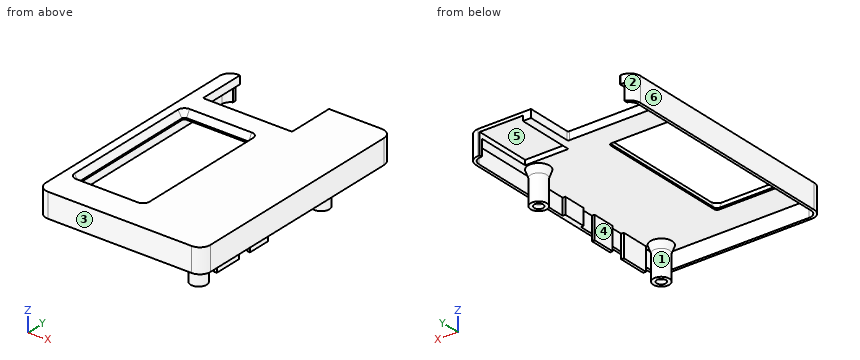
```python
from build123d import *
from OCP.BRepFilletAPI import BRepFilletAPI_MakeChamfer

# Parameters (mm, degrees)
SKETCH_1_W          = 61
SKETCH_1_H          = 90
EXTRUDE_1_DEPTH     = 3
SKETCH_3_W          = 25
SKETCH_3_H          = 51
CUT_EXTRUDE_1_DEPTH = 3
FILLET_1_R          = 1
CHAMFER_1_SIZE      = 1.4
CHAMFER_1_SIZE2     = 2.424871131
SKETCH_7_R          = 3
EXTRUDE_2_DEPTH     = 12.2
CHAMFER_2_SIZE      = 1
CHAMFER_2_SIZE2     = 2.747477419
SKETCH_8_R          = 1.3
CUT_EXTRUDE_2_DEPTH = 6
CHAMFER_3_SIZE      = 0.4
CHAMFER_3_SIZE2     = 1.098990968
SKETCH_10_W         = 1
SKETCH_10_H         = 10.4
SKETCH_10_H_2       = 8.6
EXTRUDE_3_DEPTH     = 8.5
SKETCH_11_W         = 61
SKETCH_11_H         = 90
SKETCH_11_W_2       = 59
SKETCH_11_H_2       = 88
EXTRUDE_4_DEPTH     = 6
FILLET_2_R          = 3.1
FILLET_3_R          = 3.9
CUT_EXTRUDE_3_DEPTH = 6
SKETCH_13_W         = 33
SKETCH_13_H         = 17.5
CUT_EXTRUDE_4_DEPTH = 3
FILLET_4_R          = 0.5
SKETCH_14_W         = 16
SKETCH_14_H         = 21.5
CUT_EXTRUDE_5_DEPTH = 1.8
SKETCH_15_W         = 2.5
SKETCH_15_H         = 8.6
CUT_EXTRUDE_6_DEPTH = 1


with BuildPart() as part:
    # 草图1 → 凸台-拉伸1 (new body)
    with BuildSketch(Plane.XY):
        Rectangle(SKETCH_1_W, SKETCH_1_H)
    extrude(amount=EXTRUDE_1_DEPTH)

    # 草图3 → 切除-拉伸1 (cut)
    with BuildSketch(Plane.XY.offset(3)):
        with Locations((-13.5, -7)):
            Rectangle(SKETCH_3_W, SKETCH_3_H)
    extrude(amount=-CUT_EXTRUDE_1_DEPTH, mode=Mode.SUBTRACT)

    # 圆角1
    fillet_1_edges = [part.edges().sort_by_distance(p)[0] for p in [
        (-1, -32.5, 1.5),
        (-1, 18.5, 1.5),
        (-26, 18.5, 1.5),
        (-26, -32.5, 1.5),
    ]]
    fillet(fillet_1_edges, radius=FILLET_1_R)

    # 倒角1
    chamfer_1_edges = [part.edges().sort_by_distance(p)[0] for p in [
        (-13.5, 18.5, 3),
        (-1, -7, 3),
        (-13.5, -32.5, 3),
        (-26, -7, 3),
        (-1.292893219, 18.207106781, 3),
        (-1.292893219, -32.207106781, 3),
        (-25.707106781, -32.207106781, 3),
        (-25.707106781, 18.207106781, 3),
    ]]
    chamfer_1_side = [part.faces().sort_by_distance(p)[0] for p in [
        (4.080049622, 2.115581285, 3),
    ]]
    chamfer(chamfer_1_edges, length=CHAMFER_1_SIZE, length2=CHAMFER_1_SIZE2, reference=chamfer_1_side[0])

    # 草图7 → 凸台-拉伸2 (add)
    with BuildSketch(Plane(origin=(0, 0, 0), x_dir=(-1, 0, 0), z_dir=(0, 0, -1))):
        with Locations((-24.5, -39)):
            Circle(SKETCH_7_R)
        with Locations((-24.5, 19)):
            Circle(SKETCH_7_R)
    extrude(amount=EXTRUDE_2_DEPTH)

    # 倒角2
    chamfer_2_edges = [part.edges().sort_by_distance(p)[0] for p in [
        (27.5, -39, 0),
        (27.5, 19, 0),
    ]]
    chamfer_2_side = [part.faces().sort_by_distance(p)[0] for p in [
        (3.802426395, 2.28030092, 0),
    ]]
    chamfer(chamfer_2_edges, length=CHAMFER_2_SIZE, length2=CHAMFER_2_SIZE2, reference=chamfer_2_side[0])

    # 草图8 → 切除-拉伸2 (cut)
    with BuildSketch(Plane(origin=(0, 0, -12.2), x_dir=(-1, 0, 0), z_dir=(0, 0, -1))):
        with Locations((-24.5, 19)):
            Circle(SKETCH_8_R)
        with Locations((-24.5, -39)):
            Circle(SKETCH_8_R)
    extrude(amount=-CUT_EXTRUDE_2_DEPTH, mode=Mode.SUBTRACT)

    # 倒角3: one chamfer whose edges measure the first distance from different faces: ONE call of the kernel's chamfer builder (chamfer() names one face for all edges)
    chamfer_3_edges_1 = [part.edges().sort_by_distance(p)[0] for p in [
        (25.8, 19, -12.2),
    ]]
    chamfer_3_side_1 = [part.faces().sort_by_distance(p)[0] for p in [
        (27.415147186, 19, -12.2),
    ]]
    chamfer_3_edges_2 = [part.edges().sort_by_distance(p)[0] for p in [
        (25.8, -39, -12.2),
    ]]
    chamfer_3_side_2 = [part.faces().sort_by_distance(p)[0] for p in [
        (27.415147186, -39, -12.2),
    ]]
    chamfer_3 = BRepFilletAPI_MakeChamfer(part.part.solid().wrapped)
    for e in chamfer_3_edges_1:
        chamfer_3.Add(CHAMFER_3_SIZE, CHAMFER_3_SIZE2, e.wrapped, chamfer_3_side_1[0].wrapped)  # the first distance lies on this face
    for e in chamfer_3_edges_2:
        chamfer_3.Add(CHAMFER_3_SIZE, CHAMFER_3_SIZE2, e.wrapped, chamfer_3_side_2[0].wrapped)  # the first distance lies on this face
    add(Compound.cast(chamfer_3.Shape()), mode=Mode.REPLACE)

    # 草图10 → 凸台-拉伸3 (add)
    with BuildSketch(Plane(origin=(0, 0, 0), x_dir=(-1, 0, 0), z_dir=(0, 0, -1))):
        with Locations((-29, -31.6)):
            Rectangle(SKETCH_10_W, SKETCH_10_H)
        with Locations((-29, -16.8)):
            Rectangle(SKETCH_10_W, SKETCH_10_H_2)
        with Locations((-29, -3)):
            Rectangle(SKETCH_10_W, SKETCH_10_H_2)
    extrude(amount=EXTRUDE_3_DEPTH)

    # 草图11 → 凸台-拉伸4 (add)
    with BuildSketch(Plane(origin=(0, 0, 0), x_dir=(-1, 0, 0), z_dir=(0, 0, -1))):
        Rectangle(SKETCH_11_W, SKETCH_11_H)
        Rectangle(SKETCH_11_W_2, SKETCH_11_H_2, mode=Mode.SUBTRACT)
    extrude(amount=EXTRUDE_4_DEPTH)

    # 圆角2
    fillet_2_edges = [part.edges().sort_by_distance(p)[0] for p in [
        (29.5, -44, -3),
        (29.5, 44, -3),
        (-29.5, -44, -3),
        (-29.5, 44, -3),
    ]]
    fillet(fillet_2_edges, radius=FILLET_2_R)

    # 圆角3
    fillet_3_edges = [part.edges().sort_by_distance(p)[0] for p in [
        (30.5, -45, -1.5),
        (-30.5, -45, -1.5),
        (-30.5, 45, -1.5),
        (30.5, 45, -1.5),
    ]]
    fillet(fillet_3_edges, radius=FILLET_3_R)

    # 草图12 → 切除-拉伸3 (cut)
    with BuildSketch(Plane(origin=(0, 0, -6), x_dir=(-1, 0, 0), z_dir=(0, 0, -1))):
        with BuildLine():
            Line((-26, 45), (27.6, 45))
            Line((27.6, 45), (27.6, 43.758321186))
            ThreePointArc((27.6, 43.758321186), (27.012047516, 43.938979736), (26.4, 44))
            Line((26.4, 44), (-26, 44))
            Line((-26, 44), (-26, 45))
        make_face()
    extrude(amount=-CUT_EXTRUDE_3_DEPTH, mode=Mode.SUBTRACT)

    # 草图13 → 切除-拉伸4 (cut)
    with BuildSketch(Plane.XY.offset(3)):
        with Locations((-9.5, 36.25)):
            Rectangle(SKETCH_13_W, SKETCH_13_H)
    extrude(amount=-CUT_EXTRUDE_4_DEPTH, mode=Mode.SUBTRACT)

    # 圆角4
    fillet_4_edges = [part.edges().sort_by_distance(p)[0] for p in [
        (7, 27.5, 1.5),
        (-26, 27.5, 1.5),
    ]]
    fillet(fillet_4_edges, radius=FILLET_4_R)

    # 草图14 → 切除-拉伸5 (cut)
    with BuildSketch(Plane(origin=(0, 0, 0), x_dir=(-1, 0, 0), z_dir=(0, 0, -1))):
        with Locations((-18, 34.25)):
            Rectangle(SKETCH_14_W, SKETCH_14_H)
    extrude(amount=-CUT_EXTRUDE_5_DEPTH, mode=Mode.SUBTRACT)

    # 草图15 → 切除-拉伸6 (cut)
    with BuildSketch(Plane(origin=(29.5, 0, 0), x_dir=(0, 0, -1), z_dir=(1, 0, 0))):
        with Locations((7.25, -3)):
            Rectangle(SKETCH_15_W, SKETCH_15_H)
    extrude(amount=-CUT_EXTRUDE_6_DEPTH, mode=Mode.SUBTRACT)


solid = part.part
```
Input: part model. Units: mm. Frame: model coordinates. Face numbers are marked on the shaded views. A direction names the side the tool comes from. Give positions to 0.01 mm unless a question says otherwise; leave off trailing zeros. Order: outer loops, then holes, each group sorted by start corner. A loop starts at its lowest first (then second) coordinate and runs counter-clockwise, first axis right, second up.
1. Material intervals for L1, parallel to Y at x = 24.5, z = -7.5; L2, parallel to X at y = -11, z = -1.75; L3, parallel to X at y = -29, z = -2, sorted ascending.
Derived:
L1: y = -42 to -40.3, -37.7 to -36, 16 to 17.7, 20.3 to 22
L2: x = -30.5 to -29.5, 29.5 to 30.5
L3: x = -30.5 to -29.5, 28.5 to 30.5
2. Section B-B on x = -5. Return the cut outline in (y, z), and give its area (3 significant figures).
Derived:
outline: (-45, -6) - (-44, -6) - (-44, 0) - (-32.5, 0) - (-32.5, 0.58) - (-33.9, 3) - (-45, 3) - close; (18.5, 0) - (27.5, 0) - (27.5, 3) - (19.9, 3) - (18.5, 0.58) - close
area: 67.1 mm2
3. Section C-C on x = 8. Return the cut outline in (y, z).
Derived:
outline: (-45, -6) - (-44, -6) - (-44, 0) - (45, 0) - (45, 3) - (-45, 3) - close
4. Reachability of the marked faces 4, 5 and 6 from +Z, -Z, +X, -X, +Y, -Y: full face, straight path, thin tool, end or side. Return the list, or none.
Derived:
face 4: -Z
face 5: -Z, +Y
face 6: +Z, -Z, -X, +Y, -Y
5. Mould query, pull axis Y, two halves, no side actions, for the marked faces 1, 2 and 3. Classes: released by +Y, released by -Y, zero draft, split by the parting line, or undercut.
Derived:
face 1: undercut
face 2: released by +Y
face 3: released by -Y
6. Pin query (flat end, axial travel): pin 1 (0.6 mm diameter, centred on y = 44.5, z = -4.5, fed in from +X); pin 2 (0.5 mm diameter, centred on x = 29, z = -4, fed in from +Y); pin 3 (2 mm diameter, centred on y = -15, z = -7.5, fed in from +X); pin 4 (5 mm diameter, centred on y = -1.5, z = -9, fed in from -X). Return the tip coordinate at first contact, or that it passes through.
Derived:
pin 1: stops at x = 28.97
pin 2: stops at y = 44.35
pin 3: stops at x = 29.5
pin 4: passes through
7. Section D-D on y = -39. Return the cut outline in (x, z), and give its area (3 significant figures).
Derived:
outline: (-30.5, -6) - (-29.5, -6) - (-29.5, 0) - (20.5, 0) - (21.5, -2.75) - (21.5, -12.2) - (22.8, -12.2) - (23.2, -11.1) - (23.2, -6.2) - (25.8, -6.2) - (25.8, -11.1) - (26.2, -12.2) - (27.5, -12.2) - (27.5, -2.75) - (28.5, 0) - (29.5, 0) - (29.5, -6) - (30.5, -6) - (30.5, 3) - (-30.5, 3) - close
area: 255 mm2
8. Section A-A on y = -11.5. Return the cut outline in (x, z), and give its area (3 significant figures).
Derived:
outline: (-30.5, -6) - (-29.5, -6) - (-29.5, 0) - (-26, 0) - (-26, 0.58) - (-27.4, 3) - (-30.5, 3) - close; (-1, 0) - (29.5, 0) - (29.5, -6) - (30.5, -6) - (30.5, 3) - (0.4, 3) - (-1, 0.58) - close
area: 117 mm2
